from build123d import *

# Parameters (mm, degrees)
EXTRUDE_1_DEPTH     = 25
SKETCH_2_R          = 1.5
SKETCH_2_R_2        = 4
CUT_EXTRUDE_1_DEPTH = 25
SKETCH_3_R          = 1.5
SKETCH_3_R_2        = 4
CUT_EXTRUDE_2_DEPTH = 25
FILLET_1_R          = 2


with BuildPart() as part:
    # 草图1 → 凸台-拉伸1 (new body)
    with BuildSketch(Plane(origin=(0, 0, 0), x_dir=(1, 0, 0), z_dir=(0, 1, 0))):
        Polygon((0, 0), (27.5, 0), (27.5, 44.5), (25.5, 44.5), (25.5, 2), (0, 2), align=None)
    extrude_1 = extrude(amount=EXTRUDE_1_DEPTH)

    # 草图2 → 切除-拉伸1 (cut)
    with BuildSketch(Plane(origin=(27.5, 0, 0), x_dir=(0, 0, -1), z_dir=(1, 0, 0))):
        with Locations((13.4, 12.5)):
            Circle(SKETCH_2_R)
        with Locations((32, 12.5)):
            Circle(SKETCH_2_R_2)
        with Locations((32, 19.5)):
            Circle(SKETCH_2_R)
        with Locations((39, 12.5)):
            Circle(SKETCH_2_R)
        with Locations((32, 5.5)):
            Circle(SKETCH_2_R)
        with BuildLine():
            ThreePointArc((44.5, 12.5), (40.838834765, 3.661165235), (32, 0))
            Line((32, 0), (44.5, 0))
            Line((44.5, 0), (44.5, 12.5))
        make_face()
        with BuildLine():
            ThreePointArc((32, 25), (40.838834765, 21.338834765), (44.5, 12.5))
            Line((44.5, 12.5), (44.5, 25))
            Line((44.5, 25), (32, 25))
        make_face()
        with Locations((25, 12.5)):
            Circle(SKETCH_2_R)
    cut_extrude_1 = extrude(amount=-CUT_EXTRUDE_1_DEPTH, mode=Mode.SUBTRACT)

    # 镜向1: 凸台-拉伸1, 切除-拉伸1 across plane
    add(extrude_1.mirror(Plane(origin=(0, 25, -2), x_dir=(0, 0, 1), z_dir=(1, 0, 0))))
    add(cut_extrude_1.mirror(Plane(origin=(0, 25, -2), x_dir=(0, 0, 1), z_dir=(1, 0, 0))), mode=Mode.SUBTRACT)

    # 草图3 → 切除-拉伸2 (cut)
    with BuildSketch(Plane.XY):
        with Locations((0, 19.5)):
            Circle(SKETCH_3_R)
        with Locations((7, 12.5)):
            Circle(SKETCH_3_R)
        with Locations((0, 5.5)):
            Circle(SKETCH_3_R)
        with Locations((-7, 12.5)):
            Circle(SKETCH_3_R)
        with Locations((-18.6, 12.5)):
            Circle(SKETCH_3_R)
        with Locations((0, 12.5)):
            Circle(SKETCH_3_R_2)
        with Locations((18.6, 12.5)):
            Circle(SKETCH_3_R)
    extrude(amount=-CUT_EXTRUDE_2_DEPTH, mode=Mode.SUBTRACT)

    # 圆角1
    fillet_1_edges = [part.edges().sort_by_distance(p)[0] for p in [
        (25.5, 12.5, -2),
        (27.5, 12.5, 0),
        (-25.5, 12.5, -2),
        (-27.5, 12.5, 0),
    ]]
    fillet(fillet_1_edges, radius=FILLET_1_R)


solid = part.part
Verification items for the finished model (mm, model axes). A direction names the side the tool comes from. Round coordinates to 2 decimals unless told otherwise and drop trailing zeros. Order: outer loops, then holes, each group sorted by start corner. A loop starts at its lowest first (then second) coordinate and runs counter-clockwise, first axis right, second up.
1. Section check D-D on x = 7. Record the cut outline in (y, z), then the cut area to 3 significant figures.
Final values:
outline: (0, -2) - (11, -2) - (11, 0) - (0, 0) - close; (14, -2) - (25, -2) - (25, 0) - (14, 0) - close
area: 44.0 mm2
2. Go/stop test with a flat-tipped pin: P1, Ø9, axis at x = 0, y = 12.5, coming from the -Z side. Record where the tip stops, or that it passes through.
Final values:
P1: stops at z = -2
3. Release check for a two-part mould opening along X. For faces 3 (the cylindrical face through (26.51, 5.57, -30.5)), 4 (the cylindrical face through (-24.9, 12.68, -2.57)), 5 (the cylindrical face through (-26.9, 12.68, -0.57)) record: +X half, -X half, draft (parallel to the pull), parting line (faces both ways), or undercut.
Final values:
face 3: draft
face 4: undercut
face 5: -X half
4. Section check C-C on z = -18. Record the cut outline in (x, y), then the cut area to 3 significant figures.
Final values:
outline: (-27.5, 0) - (-25.5, 0) - (-25.5, 25) - (-27.5, 25) - close; (25.5, 0) - (27.5, 0) - (27.5, 25) - (25.5, 25) - close
area: 100 mm2
5. Section check A-A on z = -13.4. Record the cut outline in (x, y), then the cut area to 3 significant figures.
Final values:
outline: (-27.5, 0) - (-25.5, 0) - (-25.5, 11) - (-27.5, 11) - close; (-27.5, 14) - (-25.5, 14) - (-25.5, 25) - (-27.5, 25) - close; (25.5, 0) - (27.5, 0) - (27.5, 11) - (25.5, 11) - close; (25.5, 14) - (27.5, 14) - (27.5, 25) - (25.5, 25) - close
area: 88.0 mm2
6. Access from +Z, -Z, +X, -X, +Y, -Y to the whole of each face (thin tool, end or side, straight path). Record for faces 1 (the flat face through (-25.5, 12, -20)), 2 (the cylindrical face through (0, 21, -1)).
Final values:
face 1: -Z, +Y, -Y
face 2: +Z, -Z
7. Thickness scan on L1, parallel to Y at x = 0, z = -0.45; L2, parallel to X at y = 4, z = -39; L3, parallel to Y at x = 26, z = -25. Record the ranges inside material, lowest first.
Final values:
L1: y = 0 to 4, 7 to 8.5, 16.5 to 18, 21 to 25
L2: x = -27.5 to -25.5, 25.5 to 27.5
L3: y = 0 to 11, 14 to 25
8. Section check B-B on x = 0. Record the cut outline in (y, z), then the cut area to 3 significant figures.
Final values:
outline: (0, -2) - (4, -2) - (4, 0) - (0, 0) - close; (7, -2) - (8.5, -2) - (8.5, 0) - (7, 0) - close; (16.5, -2) - (18, -2) - (18, 0) - (16.5, 0) - close; (21, -2) - (25, -2) - (25, 0) - (21, 0) - close
area: 22.0 mm2
